Input: part model. Units: mm. Frame: model coordinates. A direction names the side the tool comes from. Round coordinates to 2 decimals unless told otherwise and drop trailing zeros. Write each loop counter-clockwise with the first axis right and the second up, starting at its lowest first coordinate (ties: lowest second). Pieces come first, ordered by that corner, then holes. Notation, with made-up numbers: (1, 1.5) -> (23, 1.5) arc R28 ccw to (23, 28.5) -> close; hole circle Ø11 at (74, 15.25). An arc over 180 degrees is marked (long way). Use CSV: the item, a comma, the result in double quotes.
```python
from build123d import *

# Parameters (mm, degrees)
SKETCH_1_R          = 15
SKETCH_1_R_2        = 2
EXTRUDE_1_DEPTH     = 21.8
SKETCH_2_W          = 14.8
SKETCH_2_H          = 50.012193308
CUT_EXTRUDE_1_DEPTH = 61.056343124
FILLET_1_R          = 0.8
SKETCH_3_R          = 1.6
CUT_EXTRUDE_2_DEPTH = 64.191026256
SKETCH_4_W          = 18
SKETCH_4_H          = 14.8
CUT_EXTRUDE_3_DEPTH = 64.191026256
CUT_EXTRUDE_4_DEPTH = 3


with BuildPart() as part:
    # 草图1 → 凸台-拉伸1 (new body)
    with BuildSketch(Plane.XY):
        Polygon((-24.506096654, 23.006096654), (-18.506096654, 27.006096654), (18.506096654, 27.006096654), (24.506096654, 23.006096654), (24.506096654, -23.006096654), (18.506096654, -27.006096654), (-18.506096654, -27.006096654), (-24.506096654, -23.006096654), align=None)
        Circle(SKETCH_1_R, mode=Mode.SUBTRACT)
        with Locations((-20.506096654, 20.506096654)):
            Circle(SKETCH_1_R_2, mode=Mode.SUBTRACT)
        with Locations((20.506096654, 20.506096654)):
            Circle(SKETCH_1_R_2, mode=Mode.SUBTRACT)
        with Locations((20.506096654, -20.506096654)):
            Circle(SKETCH_1_R_2, mode=Mode.SUBTRACT)
        with Locations((-20.506096654, -20.506096654)):
            Circle(SKETCH_1_R_2, mode=Mode.SUBTRACT)
    extrude(amount=EXTRUDE_1_DEPTH)

    # 草图2 → 切除-拉伸1 (cut, through all)
    with BuildSketch(Plane.ZY.offset(24.506096654)):
        with Locations((10.4, 0)):
            Rectangle(SKETCH_2_W, SKETCH_2_H)
    extrude(amount=-CUT_EXTRUDE_1_DEPTH, mode=Mode.SUBTRACT)

    # 圆角1
    fillet_1_edges = [part.edges().sort_by_distance(p)[0] for p in [
        (0, -25.006096654, 17.8),
        (0, 25.006096654, 3),
        (0, -25.006096654, 3),
        (0, 25.006096654, 17.8),
    ]]
    fillet(fillet_1_edges, radius=FILLET_1_R)

    # 草图3 → 切除-拉伸2 (cut, through all)
    with BuildSketch(Plane(origin=(0, 27.006096654, 0), x_dir=(1, 0, 0), z_dir=(0, 1, 0))):
        with Locations(Location((-14, -11.8, 0), (0, 0, 270))):
            Circle(SKETCH_3_R)
        with Locations(Location((14, -11.8, 0), (0, 0, 270))):
            Circle(SKETCH_3_R)
    extrude(amount=-CUT_EXTRUDE_2_DEPTH, mode=Mode.SUBTRACT)

    # 草图4 → 切除-拉伸3 (cut, through all)
    with BuildSketch(Plane(origin=(0, 27.006096654, 0), x_dir=(1, 0, 0), z_dir=(0, 1, 0))):
        with Locations((0, -10.4)):
            Rectangle(SKETCH_4_W, SKETCH_4_H)
    extrude(amount=-CUT_EXTRUDE_3_DEPTH, mode=Mode.SUBTRACT)

    # 草图5 → 切除-拉伸4 (cut)
    with BuildSketch(Plane(origin=(0, 0, 0), x_dir=(-1, 0, 0), z_dir=(0, 0, -1))):
        with BuildLine():
            Line((-15.0260191, 9.722718241), (-12.921448383, 7.618147524))
            ThreePointArc((-12.921448383, 7.618147524), (-10.606601718, 10.606601718), (-7.618147524, 12.921448383))
            Line((-7.618147524, 12.921448383), (-9.722718241, 15.0260191))
            ThreePointArc((-9.722718241, 15.0260191), (-15.0260191, 15.0260191), (-15.0260191, 9.722718241))
        make_face()
        with BuildLine():
            Line((15.0260191, 9.722718241), (12.921448383, 7.618147524))
            ThreePointArc((12.921448383, 7.618147524), (10.606601718, 10.606601718), (7.618147524, 12.921448383))
            Line((7.618147524, 12.921448383), (9.722718241, 15.0260191))
            ThreePointArc((9.722718241, 15.0260191), (15.0260191, 15.0260191), (15.0260191, 9.722718241))
        make_face()
        with BuildLine():
            Line((9.722718241, -15.0260191), (7.618147524, -12.921448383))
            ThreePointArc((7.618147524, -12.921448383), (10.606601718, -10.606601718), (12.921448383, -7.618147524))
            Line((12.921448383, -7.618147524), (15.0260191, -9.722718241))
            ThreePointArc((15.0260191, -9.722718241), (15.0260191, -15.0260191), (9.722718241, -15.0260191))
        make_face()
        with BuildLine():
            Line((-15.0260191, -9.722718241), (-12.921448383, -7.618147524))
            ThreePointArc((-12.921448383, -7.618147524), (-10.606601718, -10.606601718), (-7.618147524, -12.921448383))
            Line((-7.618147524, -12.921448383), (-9.722718241, -15.0260191))
            ThreePointArc((-9.722718241, -15.0260191), (-15.0260191, -15.0260191), (-15.0260191, -9.722718241))
        make_face()
    extrude(amount=-CUT_EXTRUDE_4_DEPTH, mode=Mode.SUBTRACT)


solid = part.part
```
Item 1: Section query A-A on y = 0. Return the cut outline in (x, z), plus the area to 3 significant figures.
Worked answers:
outline,"(-24.51, 0) -> (-15, 0) -> (-15, 3) -> (-24.51, 3) -> close; (-24.51, 17.8) -> (-15, 17.8) -> (-15, 21.8) -> (-24.51, 21.8) -> close; (15, 0) -> (24.51, 0) -> (24.51, 3) -> (15, 3) -> close; (15, 17.8) -> (24.51, 17.8) -> (24.51, 21.8) -> (15, 21.8) -> close"
area,"133 mm²"
Item 2: Section query C-C on x = 0. Return the cut outline in (y, z), plus the area to 3 significant figures.
Worked answers:
outline,"(-27.01, 0) -> (-15, 0) -> (-15, 3) -> (-27.01, 3) -> close; (-27.01, 17.8) -> (-15, 17.8) -> (-15, 21.8) -> (-27.01, 21.8) -> close; (15, 0) -> (27.01, 0) -> (27.01, 3) -> (15, 3) -> close; (15, 17.8) -> (27.01, 17.8) -> (27.01, 21.8) -> (15, 21.8) -> close"
area,"168 mm²"
Item 3: Line query: line 1 (Z direction, x = 15, y = 17.5); line 2 (Y direction, x = -16, z = 15.75); line 3 (X direction, y = 26.25, z = 11.8). Output: solid intervals per line, ascending.
Worked answers:
line 1,"z = 0 to 3, 17.8 to 21.8"
line 2,"y = -27.01 to -25.01, 25.01 to 27.01"
line 3,"x = -19.64 to -15.6, -12.4 to -9, 9 to 12.4, 15.6 to 19.64"
Item 4: Pull-direction query (Y, two-part tool) for faces 6 (the face through (14.97, -15.08, 1.48)), 7 (the face through (24.506, 0, 1)), 8 (the face through (20.881, -25.423, 10.747)); classes: +Y half, -Y half, draft (parallel to the pull), parting line (faces both ways), or undercut.
Worked answers:
face 6,"undercut"
face 7,"draft"
face 8,"-Y half"
Item 5: Section query D-D on y = -21.5. Return the cut outline in (x, z), plus the area to 3 significant figures.
Worked answers:
outline,"(-24.51, 0) -> (-22.24, 0) -> (-22.24, 3) -> (-24.51, 3) -> close; (-24.51, 17.8) -> (-22.24, 17.8) -> (-22.24, 21.8) -> (-24.51, 21.8) -> close; (-18.77, 0) -> (18.77, 0) -> (18.77, 3) -> (-18.77, 3) -> close; (-18.77, 17.8) -> (18.77, 17.8) -> (18.77, 21.8) -> (-18.77, 21.8) -> close; (22.24, 0) -> (24.51, 0) -> (24.51, 3) -> (22.24, 3) -> close; (22.24, 17.8) -> (24.51, 17.8) -> (24.51, 21.8) -> (22.24, 21.8) -> close"
area,"294 mm²"
Item 6: Set-up query: faces 1 (the face through (15, -25.006, 10)), 2 (the face through (-20.797, -25.479, 10.747)), 3 (the face through (-8.656, 13.959, 1.479)), 4 (the face through (18.508, -20.418, 1.479)), 5 (the face through (9, 26, 11)). Return all of +Z, -Z, +X, -X, +Y, -Y with unobstructed straight access to the full face (end or side cutting, diameter ignored); none if empty.
Worked answers:
face 1,"+X, -X"
face 2,"+Z, -Z, -X, -Y"
face 3,"-Z"
face 4,"+Z, -Z"
face 5,"+Y, -Y"
Item 7: First-contact query: pin 1 Ø5 at (x, y) = (11, 12) entering from -Z; pin 2 Ø3 at (x, y) = (20.51, 20.51) entering from -Z; pin 3 Ø3 at (y, z) = (-25, 11.5) entering from +X. Flat tips, straight axial feed; report the tip coordinate or a pass-through.
Worked answers:
pin 1,"stops at z = 17.8"
pin 2,"passes through"
pin 3,"stops at x = 21.51"
Item 8: Section query B-B on z = 11.8. Give the number of separate pieces and of enclosed holes in the cut face, plus the area to 3 significant figures.
Worked answers:
separate pieces,"8"
enclosed holes,"0"
area,"62.4 mm²"
